Geometry check sheet. Reference: the model listing, model coordinates, mm. Coordinates: 2 decimals unless noted, no trailing zeros. Write each loop counter-clockwise with the first axis right and the second up, starting at its lowest first coordinate (ties: lowest second). Pieces come first, ordered by that corner, then holes. Notation, with made-up numbers: M -0.75,-33 L 41.25,-33 A27 cw 41.25,4 Z; hole C -39.5,-25.5 d11. An arc over 180 degrees is marked long. Answer as a JSON object with one key per item and string values. Group by question number.
Autodesk Inventor part; units mm, degrees
ref_plane "YZ Plane" through (0, 0, 0) normal (1, 0, 0) x (0, 1, 0)
ref_plane "XZ Plane" through (0, 0, 0) normal (0, 1, 0) x (-1, 0, 0)
ref_plane "XY Plane" through (0, 0, 0) normal (0, 0, 1) x (1, 0, 0)
sketch "Sketch1" plane through (0, 0, 0) normal (0, 0, 1) x (1, 0, 0)
  line L0 (167.1611, 130.6481) -> (167.1611, -47.4567)
  line L1 (-213.8389, -47.4567) -> (-213.8389, 130.6481)
  line L2 (-213.8389, -47.4567) -> (-150.3389, -47.4567)
  line L3 (167.1611, -47.4567) -> (103.6611, -47.4567)
  arc A0 (103.6611, -47.4567) -> (-150.3389, -47.4567) centre (-23.3389, -131.699) ccw
  line L4 (-213.8389, 130.6481) -> (-150.3389, 130.6481)
  line L5 (167.1611, 130.6481) -> (103.6611, 130.6481)
  arc A1 (-150.3389, 130.6481) -> (103.6611, 130.6481) centre (-23.3389, 214.8904) ccw
  point P0 (0, 0)
  dimension "d0" = 381
  dimension "d1" = 178.1048
  dimension "d35" = 63.5
  dimension "d36" = 63.5
  dimension "d39" = 152.4
  dimension "d40" = 63.5
  dimension "d41" = 63.5
  dimension "d42" = 152.4
extrude "Extrusion1" add sketch "Sketch1" along normal blind 6.35
fillet "Fillet1" radius 25.4 2 edges at (-150.3389, -47.4567, 3.175) (103.6611, -47.4567, 3.175)
hole "Hole1" at (-150.3389, 41.5957, 6.35) direction (0, 0, -1) diameter 63.5 end through all
hole "Hole2" at (103.6611, 41.5957, 6.35) direction (0, 0, -1) diameter 63.5 end through all
hole "Hole3" at (-201.1389, -34.7567, 6.35) direction (0, 0, -1) diameter 3.175 end through all
hole "Hole4" at (154.4611, -34.7567, 6.35) direction (0, 0, -1) diameter 3.175 end through all
pattern_linear "Rectangular Pattern4" count 7 spacing 25.4 along (0, 1, 0) of "Hole3"
pattern_linear "Rectangular Pattern5" count 7 spacing 25.4 along (0, 1, 0) of "Hole4"
properties part number "Devant - Haut Rammasse-Balle"
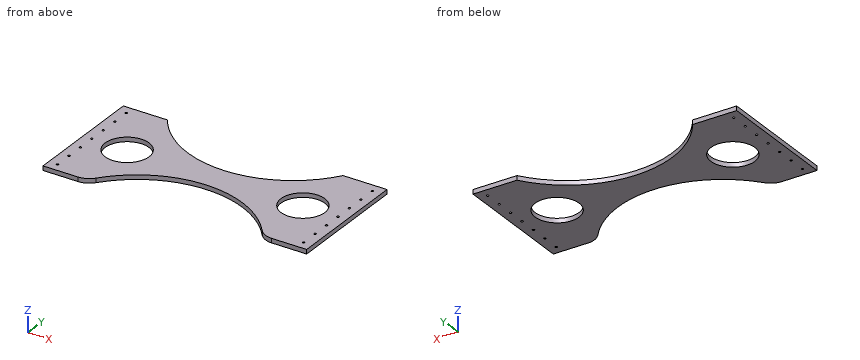
1) Section check B-B (y = 105.5). Record the cut outline in (x, z), then the cut area to 3 significant figures.
2) Section check C-C (z = 1.5). State how many separate pieces and enclosed holes the cut face has, then the cut area to 3 significant figures.
3) Go/stop test with flat-tipped pins: pin 1 Ø3 at (x, y) = (154.46, 66.84) entering from +Z; pin 2 Ø1 at (x, z) = (-130.5, 2) entering from -Y. Record where each tip stops, or that it passes through.
4) Section check A-A (x = -130.5). Record the cut outline in (y, z), then the cut area to 3 significant figures.
5) Section check D-D (x = -42). Record the cut outline in (y, z).
6) Material ranges on probe 1 along X at (y, z) = (41, 1.5); probe 2 along X at (y, z) = (31, 4.75); probe 3 along X at (y, z) = (118, 1.75), recorded low to high. Write a range as [from, to].
Entries:
{
 "1": {"outline": "M -213.84,0 L -129.45,0 L -129.45,6.35 L -213.84,6.35 Z; M 82.77,0 L 167.16,0 L 167.16,6.35 L 82.77,6.35 Z", "area": "1,070 mm^2"},
 "2": {"separate pieces": "1", "enclosed holes": "16", "area": "37,000 mm^2"},
 "3": {"pin 1": "through", "pin 2": "y = -23.83"},
 "4": {"outline": "M -23.34,0 L 16.81,0 L 16.81,6.35 L -23.34,6.35 Z; M 66.38,0 L 106.53,0 L 106.53,6.35 L 66.38,6.35 Z", "area": "510 mm^2"},
 "5": {"outline": "M 19.55,0 L 63.64,0 L 63.64,6.35 L 19.55,6.35 Z"},
 "6": {"probe 1": "[-213.84, -202.66], [-199.61, -182.08], [-118.59, 71.92], [135.41, 152.94], [155.99, 167.16]", "probe 2": "[-213.84, -180.27], [-120.41, 73.73], [133.59, 167.16]", "probe 3": "[-213.84, -202.69], [-199.59, -140.97], [94.3, 152.91], [156.01, 167.16]"}
}
